```python
from build123d import *

# Parameters (mm, degrees)
ESQUISSE1_R             = 12.5
ESQUISSE1_R_2           = 8
BOSS_EXTRU_1_DEPTH      = 200
ESQUISSE2_W             = 35
ESQUISSE2_H             = 30
BOSS_EXTRU_2_DEPTH      = 20
ESQUISSE3_R             = 2
ENL_V_MAT_EXTRU_1_DEPTH = 20


with BuildPart() as part:
    # Esquisse1 → Boss.-Extru.1 (new body)
    with BuildSketch(Plane.XY):
        Circle(ESQUISSE1_R)
        Circle(ESQUISSE1_R_2, mode=Mode.SUBTRACT)
    extrude(amount=BOSS_EXTRU_1_DEPTH)

    # Esquisse2 → Boss.-Extru.2 (add)
    with BuildSketch(Plane.XY.offset(200)):
        Rectangle(ESQUISSE2_W, ESQUISSE2_H)
    extrude(amount=BOSS_EXTRU_2_DEPTH)

    # Esquisse3 → Enlèv. mat.-Extru.1 (cut)
    with BuildSketch(Plane.XY.offset(220)):
        with Locations((5, -2)):
            Circle(ESQUISSE3_R)
        with Locations((-5, -2)):
            Circle(ESQUISSE3_R)
    extrude(amount=-ENL_V_MAT_EXTRU_1_DEPTH, mode=Mode.SUBTRACT)


solid = part.part
```
Verification items for the finished model (mm, model axes). A direction names the side the tool comes from. Round coordinates to 2 decimals unless told otherwise and drop trailing zeros. Write each loop counter-clockwise with the first axis right and the second up, starting at its lowest first coordinate (ties: lowest second). Pieces come first, ordered by that corner, then holes.
1. Section check A-A on z = 188. Enter the section's corners in (x, y), plus the area to 3 significant figures.
2. Gauge pin test, flat ends, axial feed: P1, Ø3, axis at x = 11.5, z = 98, coming from the +Y side; P2, Ø5, axis at y = 8.5, z = 165, coming from the +X side; P3, Ø5, axis at x = -11.5, z = 106, coming from the -Y side; P4, Ø3.5, axis at x = 5, y = -2, coming from the +Z side. Record the tip position at first contact, or that the pin passes through.
3. Section check B-B on x = 0. Enter the section's corners in (y, z), plus the area to 3 significant figures.
4. Section check C-C on y = -2. Enter the section's corners in (x, z), plus the area to 3 significant figures.
5. Scan lines: L1, parallel to X at y = 0.25, z = 191; L2, parallel to Y at x = 5, z = 204.25. Record each from-to range of solid material in increasing order.
6. Access from +Z, -Z, +X, -X, +Y, -Y to the whole of each face (thin tool, end or side, straight path). Record for faces 4 (the flat face through (0, 0, 200)), 5 (the cylindrical face through (-6.6, -3.2, 210.1)).
7. Draft check along X on faces 1 (the flat face through (-8, 10, 200)), 2 (the cylindrical face through (-1.73, -7.81, 98.6)), 3 (the cylindrical face through (11.923, 3.755, 98.6)). Enter one of: +X half, -X half, draft (parallel to the pull), parting line (faces both ways), or undercut.
Answer:
1. outline: circle Ø25 at (0, 0); hole circle Ø16 at (0, 0)
1. area: 290 mm2
2. P1: stops at y = 7.5
2. P2: stops at x = 10.97
2. P3: stops at y = -8.67
2. P4: passes through
3. outline: (-15, 200) - (-12.5, 200) - (-12.5, 0) - (-8, 0) - (-8, 200) - (8, 200) - (8, 0) - (12.5, 0) - (12.5, 200) - (15, 200) - (15, 220) - (-15, 220) - close
3. area: 2,400 mm2
4. outline: (-17.5, 200) - (-12.34, 200) - (-12.34, 0) - (-7.75, 0) - (-7.75, 200) - (-7, 200) - (-7, 220) - (-17.5, 220) - close; (-3, 200) - (3, 200) - (3, 220) - (-3, 220) - close; (7, 200) - (7.75, 200) - (7.75, 0) - (12.34, 0) - (12.34, 200) - (17.5, 200) - (17.5, 220) - (7, 220) - close
4. area: 2,380 mm2
5. L1: x = -12.5 to -8, 8 to 12.5
5. L2: y = -15 to -4, 0 to 15
6. face 4: -Z
6. face 5: +Z, -Z
7. face 1: draft
7. face 2: undercut
7. face 3: parting line
